from build123d import *

# Parameters (mm, degrees)
BOSS_EXTRUDE1_DEPTH = 30
BOSS_EXTRUDE2_DEPTH = 30
FILLET1_R           = 7
CUT_EXTRUDE1_DEPTH  = 91


with BuildPart() as part:
    # Sketch1 → Boss-Extrude1 (new body, symmetric)
    with BuildSketch(Plane(origin=(0, 0, 0), x_dir=(0, 0, -1), z_dir=(1, 0, 0))):
        Polygon((-20, 0), (20, 0), (20, 5), (45, 5), (45, 15), (-45, 15), (-45, 5), (-20, 5), align=None)
    extrude(amount=BOSS_EXTRUDE1_DEPTH, both=True)

    # Sketch4 → Boss-Extrude2 (add, symmetric)
    with BuildSketch(Plane(origin=(0, 0, 0), x_dir=(0, 0, -1), z_dir=(1, 0, 0))):
        with BuildLine():
            Line((30, 15), (30, 43))
            ThreePointArc((30, 43), (26.537038068, 49.040642491), (19.574468085, 49.104566414))
            ThreePointArc((19.574468085, 49.104566414), (0, 43.987803064), (-19.574468085, 49.104566414))
            ThreePointArc((-19.574468085, 49.104566414), (-26.537038068, 49.040642491), (-30, 43))
            Line((-30, 43), (-30, 15))
            Line((-30, 15), (30, 15))
        make_face()
    extrude(amount=BOSS_EXTRUDE2_DEPTH, both=True)

    # Fillet1
    fillet1_edges = [part.edges().sort_by_distance(p)[0] for p in [
        (0, 15, 30),
        (0, 15, -30),
    ]]
    fillet(fillet1_edges, radius=FILLET1_R)

    # Sketch5 → Cut-Extrude1 (cut, through all)
    with BuildSketch(Plane.XY.offset(45)):
        with BuildLine():
            ThreePointArc((-7.72740661, 46.058355425), (-6.794626723, 48.210722397), (-5.277640382, 50))
            Line((-5.277640382, 50), (-30, 50))
            Line((-30, 50), (-30, 15))
            Line((-30, 15), (-26.792045696, 15))
            ThreePointArc((-26.792045696, 15), (-18.26938569, 17.893053236), (-13.269084128, 25.376533369))
            Line((-13.269084128, 25.376533369), (-7.72740661, 46.058355425))
        make_face()
        with BuildLine():
            ThreePointArc((5.277640382, 50), (6.794626723, 48.210722397), (7.72740661, 46.058355425))
            Line((7.72740661, 46.058355425), (13.269084128, 25.376533369))
            ThreePointArc((13.269084128, 25.376533369), (18.26938569, 17.893053236), (26.792045696, 15))
            Line((26.792045696, 15), (30, 15))
            Line((30, 15), (30, 50))
            Line((30, 50), (5.277640382, 50))
        make_face()
    extrude(amount=-CUT_EXTRUDE1_DEPTH, mode=Mode.SUBTRACT)


solid = part.part
Design review of the part built by this model. Coordinates are the model's own, in mm. A direction names the side the tool comes from. Give positions to 0.01 mm unless a question says otherwise; leave off trailing zeros. Write each loop counter-clockwise with the first axis right and the second up, starting at its lowest first coordinate (ties: lowest second). Pieces come first, ordered by that corner, then holes. Notation, with made-up numbers: M -11,52 L 4,52 A30 ccw 4,87 Z; hole C 62.25,33.25 d3. An arc over 180 degrees is marked long. Return JSON: item names as keys, results as strings. Group by question number.
Item 1: Tool access review of faces 5 (the flat face through (-30, 9, 1)), 6 (the flat face through (10.46, 35.86, 0.42)), 7 (the flat face through (0, 5, 33)), 8 (the flat face through (0, 2, -20)), 9 (the flat face through (0, 32, -30)): name each direction out of +Z, -Z, +X, -X, +Y, -Y from which nothing blocks a thin tool from reaching the whole face with its end or side.
Item 2: Take a section at A-A (x = 3). Give the boundary of the cut face in (y, z).
Item 3: The part is to be moulded in two halves that separate along Z. For faces 1 (the flat face through (30, 9, 1)), 2 (the flat face through (0, 10, 45)), 3 (the flat face through (0, 10, -45)), 4 (the cylindrical face through (0.12, 49.09, 26.45)), say which applies: pulls with the +Z half, pulls with the -Z half, needs draft (parallel to the pull), parting line crosses it, or undercut.
Item 4: Take a section at B-B (z = -18). Give the boundary of the cut face in (x, y).
Item 5: Take a section at C-C (y = 40). Give the boundary of the cut face in (x, z).
Item 6: Take a section at D-D (x = -22). Give the boundary of the cut face in (y, z), plus the area to 3 significant figures.
Item 7: Wall thickness on line 1 along Z through (x, y) = (-2, 33); line 2 along Z through (x, y) = (-6, 47); line 3 along Y through (x, z) = (19.5, 39): over which ranges is each line inside the solid? List them lowest first.
Item 8: Clearance check with flat-ended pins moving along their axes: pin 1 Ø4 at (y, z) = (33, -7.5) entering from +X; pin 2 Ø10.5 at (x, y) = (-2.5, 32) entering from +Z; pin 3 Ø8 at (y, z) = (21.5, -14) entering from +X. State where each tip first meets the part, or that it passes through.
Return value:
{
 "1": {"face 5": "+Z, -Z, -X, +Y, -Y", "face 6": "+Z, -Z, +X, +Y", "face 7": "+Z, +X, -X, -Y", "face 8": "-Z, +X, -X, -Y", "face 9": "-Z, +X, -X, +Y"},
 "2": {"outline": "M 0,-20 L 5,-20 L 5,-45 L 15,-45 L 15,-37 A7 cw 22,-30 L 43,-30 A7 ccw 49.1,-19.57 A40 cw 49.1,19.57 A7 ccw 43,30 L 22,30 A7 cw 15,37 L 15,45 L 5,45 L 5,20 L 0,20 Z"},
 "3": {"face 1": "needs draft", "face 2": "pulls with the +Z half", "face 3": "pulls with the -Z half", "face 4": "undercut"},
 "4": {"outline": "M -30,0 L 30,0 L 30,15 L 26.79,15 A14 cw 13.27,25.38 L 7.73,46.06 A8 ccw 6.76,48.27 L -6.76,48.27 A8 ccw -7.73,46.06 L -13.27,25.38 A14 cw -26.79,15 L -30,15 Z"},
 "5": {"outline": "M -9.35,-30 L 9.35,-30 L 9.35,30 L -9.35,30 Z"},
 "6": {"outline": "M 0,-20 L 5,-20 L 5,-45 L 15,-45 L 15,-37 A7 cw 15.85,-33.66 L 15.85,33.66 A7 cw 15,37 L 15,45 L 5,45 L 5,20 L 0,20 Z", "area": "1,160 mm2"},
 "7": {"line 1": "z = -30 to 30", "line 2": "z = -28.74 to -15.23, 15.23 to 28.74", "line 3": "y = 5 to 15"},
 "8": {"pin 1": "stops at x = 11.76", "pin 2": "stops at z = 30", "pin 3": "stops at x = 18.81"}
}
